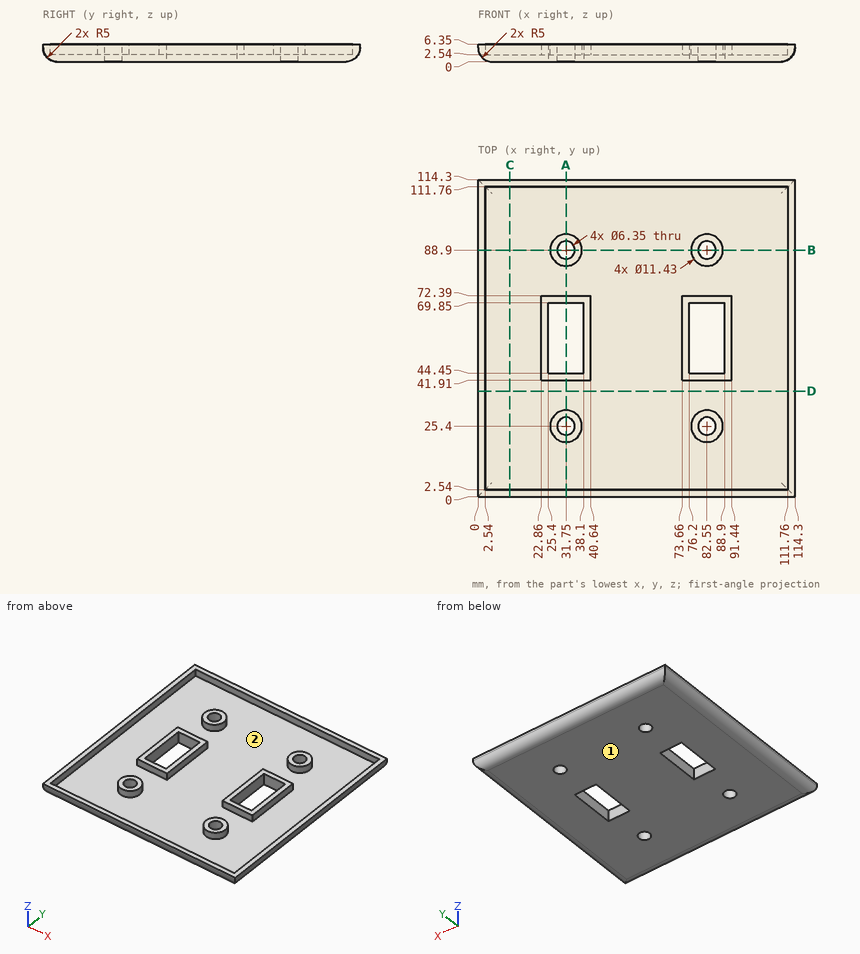
Can you work these out from the drawing? Everything is in mm from the part's minimum corner. A direction names the side the tool comes from. Give positions to 0.01 mm unless a question says otherwise; leave off trailing zeros. Loops run counter-clockwise (first coordinate to the right, second up) from the corner with the lowest first, then second, coordinate; pieces in that order, holes last. Notation, with made-up numbers: (57, 26) - (68, 26) arc R24 cw to (68, 64) - close; hole circle Ø5 at (53, 37). An arc over 180 degrees is marked (long way). Answer as a JSON object with one key per item and string values.
Q1. Imagine slicing it at A-A on x = 31.75. Give the number of separate pieces and of enclosed holes in the cut face, plus the area to 3 significant figures.
Geometry says:
{"separate pieces": "4", "enclosed holes": "0", "area": "260 mm²"}
Q2. If I drill on L1, parallel to Y at x = 52, z = 6.25; L2, parallel to X at y = 62, z = 3.5; L3, parallel to X at y = 50, z = 3, over which ranges is the centre line in solid material (lowest first)?
Geometry says:
{"L1": "0 to 2.54, 111.76 to 114.3", "L2": "0.23 to 2.54, 22.86 to 25.4, 38.1 to 40.64, 73.66 to 76.2, 88.9 to 91.44, 111.76 to 114.07", "L3": "0.42 to 2.54, 22.86 to 25.4, 38.1 to 40.64, 73.66 to 76.2, 88.9 to 91.44, 111.76 to 113.88"}
Q3. Will these pins go through, and if not, where does the flat tip stop? P1, Ø2, axis at y = 99.5, z = 3, coming from the +X side; P2, Ø1.9, axis at x = 85.5, z = 2.5, coming from the +Y side; P3, Ø4, axis at x = 62, y = 60.5, coming from the +Z side; P4, Ø5, axis at x = 82.55, y = 25.4, coming from the -Z side.
Geometry says:
{"P1": "x = 114.2", "P2": "y = 114.05", "P3": "z = 2.54", "P4": "through"}
Q4. Imagine slicing it at C-C on x = 11.5. Write out the boundary of the cut face in (y, z).
Geometry says:
{"outline": "(0, 5) arc R5 ccw to (5, 0) - (109.3, 0) arc R5 ccw to (114.3, 5) - (114.3, 6.35) - (111.76, 6.35) - (111.76, 2.54) - (2.54, 2.54) - (2.54, 6.35) - (0, 6.35) - close"}
Q5. Imagine slicing it at B-B on y = 88.9. Write out the boundary of the cut face in (x, z) (3 decimals).
Geometry says:
{"outline": "(0, 5) arc R5 ccw to (5, 0) - (28.575, 0) - (28.575, 6.35) - (26.035, 6.35) - (26.035, 2.54) - (2.54, 2.54) - (2.54, 6.35) - (0, 6.35) - close; (34.925, 0) - (79.375, 0) - (79.375, 6.35) - (76.835, 6.35) - (76.835, 2.54) - (37.465, 2.54) - (37.465, 6.35) - (34.925, 6.35) - close; (85.725, 0) - (109.3, 0) arc R5 ccw to (114.3, 5) - (114.3, 6.35) - (111.76, 6.35) - (111.76, 2.54) - (88.265, 2.54) - (88.265, 6.35) - (85.725, 6.35) - close"}
Q6. Which directions (+Z, -Z, +X, -X, +Y, -Y) give clear straight access to the entire face, cutting with the end or side of a thin tool? Please do the marked faces 1 and 2.
Geometry says:
{"face 1": "-Z, +X, -X, +Y, -Y", "face 2": "+Z"}
